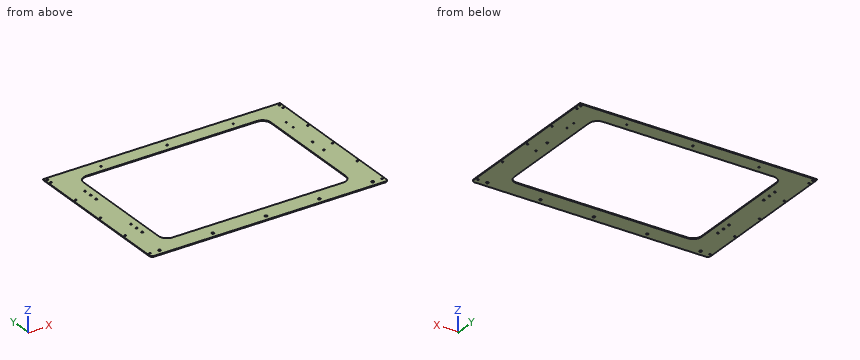
from build123d import *

# Parameters (mm, degrees)
SKETCH1_W            = 856
SKETCH1_H            = 543.9
MAINFRONT_DEPTH      = 3
SKETCH2_W            = 676
SKETCH2_H            = 463.9
DOORCUT_DEPTH        = 4
DOORROUNDINTERNAL_R  = 30
SKETCH3_W            = 856
SKETCH3_H            = 40
BOTTOMMOUNT_DEPTH    = 3
M8_CLEARANCE_HOLE1_D = 9
LPATTERN1_COUNT      = 5
LPATTERN1_PITCH      = 192.5
M5_CLEARANCE_HOLE1_D = 5.5
LPATTERN2_COUNT      = 5
LPATTERN2_PITCH      = 133.475
MIRROR1_COPY_1_D     = 5.5
MIRROR1_COPY_2_D     = 5.5
MIRROR1_COPY_3_D     = 5.5
MIRROR1_COPY_4_D     = 5.5
M5_CLEARANCE_HOLE2_D = 5.5
LPATTERN3_COUNT      = 2
LPATTERN3_PITCH      = 838
M6_CLEARANCE_HOLE1_D = 6.6
FILLET1_R            = 10
M4_CLEARANCE_HOLE1_D = 4.5
M6_CLEARANCE_HOLE2_D = 6.6
M5_CLEARANCE_HOLE3_D = 5.8


with BuildPart() as part:
    # Sketch1 → MainFront (new body)
    with BuildSketch(Plane.XY):
        with Locations((428, 271.95)):
            Rectangle(SKETCH1_W, SKETCH1_H)
    extrude(amount=MAINFRONT_DEPTH)

    # Sketch2 → DoorCut (cut, through all)
    with BuildSketch(Plane.XY.offset(3)):
        with Locations((428, 256.95)):
            Rectangle(SKETCH2_W, SKETCH2_H)
    extrude(amount=-DOORCUT_DEPTH, mode=Mode.SUBTRACT)

    # DoorRoundInternal
    doorroundinternal_edges = [part.edges().sort_by_distance(p)[0] for p in [
        (766, 488.9, 1.5),
        (766, 25, 1.5),
        (90, 25, 1.5),
        (90, 488.9, 1.5),
    ]]
    fillet(doorroundinternal_edges, radius=DOORROUNDINTERNAL_R)

    # Sketch3 → BottomMount (add)
    with BuildSketch(Plane.XY.offset(3)):
        with Locations((428, -20)):
            Rectangle(SKETCH3_W, SKETCH3_H)
    extrude(amount=-BOTTOMMOUNT_DEPTH)

    # M8 Clearance Hole1 (through all)
    with Locations(Plane.XY.offset(3)):
        with Locations((43, -20)):
            m8_clearance_hole1 = Hole(M8_CLEARANCE_HOLE1_D / 2)

    # LPattern1: M8 Clearance Hole1 ×5
    with Locations(*[(i * LPATTERN1_PITCH, 0, 0) for i in range(1, LPATTERN1_COUNT)]):
        add(m8_clearance_hole1, mode=Mode.SUBTRACT)

    # M5 Clearance Hole1 (through all)
    with Locations(Plane.XY.offset(3)):
        with Locations((9, -20)):
            m5_clearance_hole1 = Hole(M5_CLEARANCE_HOLE1_D / 2)

    # LPattern2: M5 Clearance Hole1 ×5
    with Locations(*[(0, i * LPATTERN2_PITCH, 0) for i in range(1, LPATTERN2_COUNT)]):
        add(m5_clearance_hole1, mode=Mode.SUBTRACT)

    # Mirror1: M5 Clearance Hole1 across plane
    add(m5_clearance_hole1.mirror(Plane(origin=(428, 0, 0), x_dir=(0, 0, 1), z_dir=(1, 0, 0))), mode=Mode.SUBTRACT)

    # Mirror1 copy 1 (through all)
    with Locations(Plane(origin=(856, 133.475, 3), x_dir=(-1, 0, 0), z_dir=(0, 0, 1))):
        with Locations((9, 20)):
            Hole(MIRROR1_COPY_1_D / 2)

    # Mirror1 copy 2 (through all)
    with Locations(Plane(origin=(856, 266.95, 3), x_dir=(-1, 0, 0), z_dir=(0, 0, 1))):
        with Locations((9, 20)):
            Hole(MIRROR1_COPY_2_D / 2)

    # Mirror1 copy 3 (through all)
    with Locations(Plane(origin=(856, 400.425, 3), x_dir=(-1, 0, 0), z_dir=(0, 0, 1))):
        with Locations((9, 20)):
            Hole(MIRROR1_COPY_3_D / 2)

    # Mirror1 copy 4 (through all)
    with Locations(Plane(origin=(856, 533.9, 3), x_dir=(-1, 0, 0), z_dir=(0, 0, 1))):
        with Locations((9, 20)):
            Hole(MIRROR1_COPY_4_D / 2)

    # M5 Clearance Hole2 (through all)
    with Locations(Plane.XY.offset(3)):
        with Locations((9, 533.9)):
            m5_clearance_hole2 = Hole(M5_CLEARANCE_HOLE2_D / 2)

    # LPattern3: M5 Clearance Hole2 ×2
    with Locations(*[(i * LPATTERN3_PITCH, 0, 0) for i in range(1, LPATTERN3_COUNT)]):
        add(m5_clearance_hole2, mode=Mode.SUBTRACT)

    # M6 Clearance Hole1 (through all)
    with Locations(Plane.XY.offset(3)):
        with Locations((802, 286.95), (802, 226.95)):
            Hole(M6_CLEARANCE_HOLE1_D / 2)

    # Fillet1
    fillet1_edges = [part.edges().sort_by_distance(p)[0] for p in [
        (0, -40, 1.5),
        (856, -40, 1.5),
    ]]
    fillet(fillet1_edges, radius=FILLET1_R)

    # M4 Clearance Hole1 (through all)
    with Locations(Plane.XY.offset(3)):
        with Locations((804.180642757, 432.408967428), (804.180642757, 396.408967428)):
            Hole(M4_CLEARANCE_HOLE1_D / 2)

    # M6 Clearance Hole2 (through all)
    with Locations(Plane.XY.offset(3)):
        with Locations((63, 410.9), (63, 380.9), (63, 350.9)):
            m6_clearance_hole2 = Hole(M6_CLEARANCE_HOLE2_D / 2)

    # Mirror2: M6 Clearance Hole2 across plane
    add(m6_clearance_hole2.mirror(Plane.ZX.offset(256.95)), mode=Mode.SUBTRACT)

    # M5 Clearance Hole3 (through all)
    with Locations(Plane.XY.offset(3)):
        with Locations((189, 513.9), (428, 513.9), (667, 513.9)):
            Hole(M5_CLEARANCE_HOLE3_D / 2)


solid = part.part
Verification items for the finished model (mm, model axes). Give positions to 0.01 mm unless a question says otherwise; leave off trailing zeros. Loops run counter-clockwise (first coordinate to the right, second up) from the corner with the lowest first, then second, coordinate; pieces in that order, holes last.
1) Thickness scan on line 1 along X through (y, z) = (246.95, 0.95); line 2 along X through (y, z) = (328, 2.4); line 3 along Y through (x, z) = (203, 2.3). Record the ranges inside material, lowest first.
2) Sectioned sample at A-A, the plane x = 131. Enter the section's corners in (y, z), then the cut area to 3 significant figures.
3) Sectioned sample at B-B, the plane z = 1.3. Count the separate pieces of the cut face and the enclosed holes in it, then the cut area to 3 significant figures.
4) Depth check by flat-ended pin: pin 1 Ø8.5 at (x, y) = (802, 286.95) entering from +Z. Enter the tip coordinate at first touch or a pass-through.
Answers:
1. line 1: x = 0 to 6.25, 11.75 to 90, 766 to 844.25, 849.75 to 856
1. line 2: x = 0 to 90, 766 to 856
1. line 3: y = -40 to 25, 488.9 to 543.9
2. outline: (-40, 0) - (25, 0) - (25, 3) - (-40, 3) - close; (488.9, 0) - (543.9, 0) - (543.9, 3) - (488.9, 3) - close
2. area: 360 mm2
3. separate pieces: 1
3. enclosed holes: 31
3. area: 186,000 mm2
4. pin 1: stops at z = 3
